Source: CAD feature listing. Evaluate the final solid. Frame: model axes, mm. Face numbers are marked on the shaded views. A direction names the side the tool comes from. Coordinates: 2 decimals unless noted, no trailing zeros. Write each loop counter-clockwise with the first axis right and the second up, starting at its lowest first coordinate (ties: lowest second). Pieces come first, ordered by that corner, then holes. Notation, with made-up numbers: M 71.5,-15.5 L 108.5,-15.5 A24 cw 108.5,0.5 Z; hole C -30,55 d9. An arc over 180 degrees is marked long. Write item = value, one per line. Start each with the question number.
1. Line query: line 1 along X through (y, z) = (-60.5, 27.5); line 2 along Y through (x, z) = (-35.5, 30); line 3 along Y through (x, z) = (-111.5, 12). Output: solid intervals per line, ascending.
2. Pull-direction query (Y, two-part tool) for the marked faces 1, 2 and 3; classes: pulls with the +Y half, pulls with the -Y half, needs draft (parallel to the pull), parting line crosses it, or undercut.
3. Section query B-B (y = -106.5). Output: boundary loops of the cut face in (x, z), then the cut area to 3 significant figures.
4. Section query A-A (z = 48). Output: boundary loops of the cut face in (x, y).
5. Section query D-D (z = 24.5). Give the number of separate pieces and of enclosed holes in the cut face, then the cut area to 3 significant figures.
6. Section query C-C (x = -15). Output: boundary loops of the cut face in (y, z).
7. Access query for the marked faces 4 and 5. Directions: +Z, -Z, +X, -X, +Y, -Y. A direction counts if a zero-diameter tool reaches every point of the face in a straight line with its end or side. Return the directions, or none.
8. Pin query (flat end, axial travel): pin 1 Ø4 at (x, y) = (-122, -42.5) entering from -Z; pin 2 Ø1 at (x, y) = (-91.5, -23) entering from -Z; pin 3 Ø19 at (x, y) = (-140, -95) entering from -Z. Return the tip coordinate at first contact, or that it passes through.
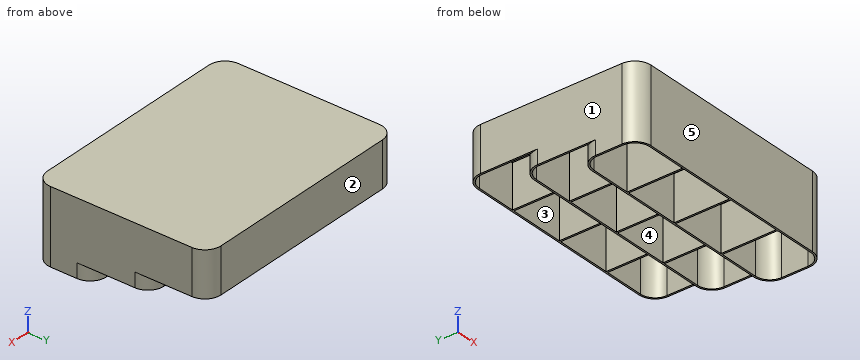
```python
from build123d import *

# Parameters (mm, degrees)
F0_W     = 160
F0_H     = 120
F0_W_2   = 38.2
F0_H_2   = 38.2
F0_W_3   = 38.8
F0_H_3   = 38.8
F1_DEPTH = 50
F2_W     = 160
F2_H     = 120
F3_DEPTH = 1.2
F5_DEPTH = 160.001
F7_DEPTH = 158.8
F8_R     = 10
F9_R     = 11.2
F10_R    = 10
F11_R    = 11.2
F11_R_2  = 11.19999


# Not quite as in the source:
# - a fillet or chamfer is up to 0.001 mm smaller than in the source, because OpenCascade refuses the exact size


with BuildPart() as f1:
    # F0 (on Top) → F1 (new body)
    with BuildSketch(Plane.XY):
        with Locations((-80, -60)):
            Rectangle(F0_W, F0_H)
        with Locations((-139.7, -99.7)):
            Rectangle(F0_W_2, F0_H_2, mode=Mode.SUBTRACT)
        with Locations((-100, -99.7)):
            Rectangle(F0_W_3, F0_H_2, mode=Mode.SUBTRACT)
        with Locations((-60, -99.7)):
            Rectangle(F0_W_3, F0_H_2, mode=Mode.SUBTRACT)
        with Locations((-20.3, -99.7)):
            Rectangle(F0_W_2, F0_H_2, mode=Mode.SUBTRACT)
        with Locations((-139.7, -60)):
            Rectangle(F0_W_2, F0_H_3, mode=Mode.SUBTRACT)
        with Locations((-100, -60)):
            Rectangle(F0_W_3, F0_H_3, mode=Mode.SUBTRACT)
        with Locations((-139.7, -20.3)):
            Rectangle(F0_W_2, F0_H_2, mode=Mode.SUBTRACT)
        with Locations((-100, -20.3)):
            Rectangle(F0_W_3, F0_H_2, mode=Mode.SUBTRACT)
        with Locations((-60, -60)):
            Rectangle(F0_W_3, F0_H_3, mode=Mode.SUBTRACT)
        with Locations((-20.3, -60)):
            Rectangle(F0_W_2, F0_H_3, mode=Mode.SUBTRACT)
        with Locations((-60, -20.3)):
            Rectangle(F0_W_3, F0_H_2, mode=Mode.SUBTRACT)
        with Locations((-20.3, -20.3)):
            Rectangle(F0_W_2, F0_H_2, mode=Mode.SUBTRACT)
    extrude(amount=F1_DEPTH)

    # F2 (on face) → F3 (join)
    with BuildSketch(Plane.XY.offset(50)):
        with Locations((-80, -60)):
            Rectangle(F2_W, F2_H)
    extrude(amount=F3_DEPTH)

    # F4 (on face) → F5 (cut, through all)
    with BuildSketch(Plane(origin=(-160, 0, 0), x_dir=(0, -1, 0), z_dir=(-1, 0, 0))):
        Polygon((79.4, 0), (79.4, 10), (39.4, 10), (39.4, 20), (0, 20), (0, 0), align=None)
    extrude(amount=-F5_DEPTH, mode=Mode.SUBTRACT)

    # F6 (on face) → F7 (join, through all)
    with BuildSketch(Plane(origin=(-160, 0, 0), x_dir=(0, -1, 0), z_dir=(-1, 0, 0))):
        Polygon((40.6, 50), (40.6, 41.2), (79.4, 41.2), (79.4, 31.2), (118.8, 31.2), (118.8, 50), align=None)
    extrude(amount=-F7_DEPTH)

    # F8
    f8_edges = [f1.edges().sort_by_distance(p)[0] for p in [
        (-1.2, -118.8, 15.6),
        (-1.2, -1.2, 35),
        (-158.8, -118.8, 15.6),
        (-158.8, -1.2, 35),
    ]]
    fillet(f8_edges, radius=F8_R)

    # F9
    f9_edges = [f1.edges().sort_by_distance(p)[0] for p in [
        (-160, 0, 35.6),
        (0, 0, 35.6),
        (0, -120, 25.6),
        (-160, -120, 25.6),
    ]]
    fillet(f9_edges, radius=F9_R)

    # F10
    f10_edges = [f1.edges().sort_by_distance(p)[0] for p in [
        (-158.8, -80.6, 15.6),
        (-158.8, -40.6, 25.6),
        (-1.2, -40.6, 25.6),
        (-1.2, -80.6, 15.6),
    ]]
    fillet(f10_edges, radius=F10_R)

    # F11 (call 1 of 4: OpenCascade refuses the feature's edges together)
    f11_edges = [f1.edges().sort_by_distance(p)[0] for p in [
        (-160, -79.4, 5),
    ]]
    fillet(f11_edges, radius=F11_R)

    # F11#2 (call 2 of 4)
    f11_2_edges = [f1.edges().sort_by_distance(p)[0] for p in [
        (-160, -39.4, 15),
    ]]
    fillet(f11_2_edges, radius=F11_R)

    # F11#3 (call 3 of 4) (radius 11.2 in the source; OpenCascade refuses exactly that, so slightly less here)
    f11_3_edges = [f1.edges().sort_by_distance(p)[0] for p in [
        (0, -79.4, 5),
    ]]
    fillet(f11_3_edges, radius=F11_R_2)

    # F11#4 (call 4 of 4)
    f11_4_edges = [f1.edges().sort_by_distance(p)[0] for p in [
        (0, -39.4, 15),
    ]]
    fillet(f11_4_edges, radius=F11_R)


solid = f1.part
```
Results are:
q1.line_1 = -160 to -158.8, -120.6 to -119.4, -80.6 to -79.4, -40.6 to -39.4, -1.2 to 0
q1.line_2 = -120 to -118.8, -80.6 to -79.4, -40.6 to -39.4, -1.2 to 0
q1.line_3 = -120 to -118.8, -80.6 to -79.4, -40.6 to -39.4
q2.face_1 = needs draft
q2.face_2 = pulls with the +Y half
q2.face_3 = undercut
q3.outline = M -160,0 L -158.8,0 L -158.8,31.2 L -120.6,31.2 L -120.6,0 L -119.4,0 L -119.4,31.2 L -80.6,31.2 L -80.6,0 L -79.4,0 L -79.4,31.2 L -40.6,31.2 L -40.6,0 L -39.4,0 L -39.4,31.2 L -1.2,31.2 L -1.2,0 L 0,0 L 0,51.2 L -160,51.2 Z
q3.area = 3,390 mm^2
q4.outline = M -160,-108.8 A11.2 ccw -148.8,-120 L -11.2,-120 A11.2 ccw 0,-108.8 L 0,-11.2 A11.2 ccw -11.2,0 L -148.8,0 A11.2 ccw -160,-11.2 Z; hole M -158.8,-45.56 A11.2 cw -148.8,-39.4 L -120.6,-39.4 L -120.6,-1.2 L -148.8,-1.2 A10 ccw -158.8,-11.2 Z; hole M -119.4,-39.4 L -80.6,-39.4 L -80.6,-1.2 L -119.4,-1.2 Z; hole M -79.4,-39.4 L -40.6,-39.4 L -40.6,-1.2 L -79.4,-1.2 Z; hole M -39.4,-39.4 L -11.2,-39.4 A11.2 cw -1.2,-45.56 L -1.2,-11.2 A10 ccw -11.2,-1.2 L -39.4,-1.2 Z
q5.separate_pieces = 1
q5.enclosed_holes = 12
q5.area = 1,450 mm^2
q6.outline = M -120,0 L -118.8,0 L -118.8,31.2 L -80.6,31.2 L -80.6,0 L -79.4,0 L -79.4,41.2 L -40.6,41.2 L -40.6,10 L -39.4,10 L -39.4,50 L -1.2,50 L -1.2,20 L 0,20 L 0,51.2 L -120,51.2 Z
q7.face_4 = -Z
q7.face_5 = +Z, -Z, +X, -X, -Y
q8.pin_1 = 10
q8.pin_2 = 50
q8.pin_3 = 31.2
